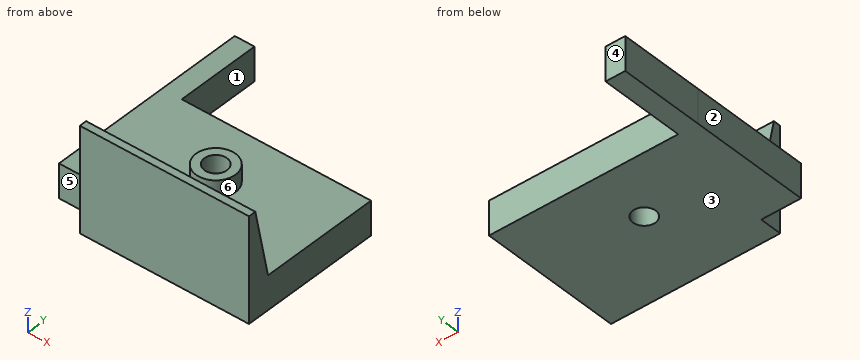
from build123d import *

# Parameters (mm, degrees)
F0_W      = 3.500263
F0_H      = 15
F1_DEPTH  = 6
F2_R      = 3.5
F2_R_2    = 2
F3_DEPTH  = 3
F3_FACE_R = 2
F4_DEPTH  = 25
F6_DEPTH  = 30


with BuildPart() as f1:
    # F0 (on Top) → F1 (new body)
    with BuildSketch(Plane.XY):
        with Locations((-35.299869, 28.75)):
            Rectangle(F0_W, F0_H)
        Polygon((-37.05, 0), (0, 0), (0, 21.25), (-33.549737, 21.25), (-37.05, 21.25), align=None)
    extrude(amount=F1_DEPTH)

    # F2 (on face) → F3 (join)
    with BuildSketch(Plane.XY.offset(6)):
        with Locations((-18.5, 10.75)):
            Circle(F2_R)
        with Locations((-18.5, 10.75)):
            Circle(F2_R_2, mode=Mode.SUBTRACT)
    extrude(amount=F3_DEPTH)

    # F3_face (on face) → F4 (cut)
    with BuildSketch(Plane(origin=(-18.5, 10.75, 6), x_dir=(1, 0, 0), z_dir=(0, 0, 1))):
        Circle(F3_FACE_R)
    extrude(amount=-F4_DEPTH, mode=Mode.SUBTRACT)

    # F5 (on face) → F6 (join)
    with BuildSketch(Plane.YZ):
        Polygon((-3.914129, 0), (0, 0), (0, 6), (-2.612495, 18.507209), (-3.914129, 18.507209), align=None)
    extrude(amount=-F6_DEPTH)


solid = f1.part
Check sheet for the modelled part. Datum: model origin and axes. Units: mm. Face numbers are marked on the shaded views. A direction names the side the tool comes from. Give positions to 0.01 mm unless a question says otherwise; leave off trailing zeros. Write each loop counter-clockwise with the first axis right and the second up, starting at its lowest first coordinate (ties: lowest second). Pieces come first, ordered by that corner, then holes. Notation, with made-up numbers: (38.5, 68.25) -> (70.5, 68.25) arc R15 ccw to (70.5, 95.25) -> close; hole circle Ø2 at (-31.5, -26). An arc over 180 degrees is marked (long way). Write item = value, one per line.
Item 1: Sectioned sample at B-B on y = 10.75. Record the boundary of the cut face in (x, z).
Output:
outline = (-37.05, 0) -> (-20.5, 0) -> (-20.5, 9) -> (-22, 9) -> (-22, 6) -> (-37.05, 6) -> close; (-16.5, 0) -> (0, 0) -> (0, 6) -> (-15, 6) -> (-15, 9) -> (-16.5, 9) -> close
Item 2: Release check for a two-part mould opening along Y. For the marked faces 3, 4, 5 and 6 record: +Y half, -Y half, draft (parallel to the pull), parting line (faces both ways), or undercut.
Output:
face_3 = draft
face_4 = +Y half
face_5 = -Y half
face_6 = undercut
Item 3: Scan lines: probe 1 along Y at (x, z) = (-18.5, 1.6); probe 2 along Z at (x, y) = (-32.5, 15.5); probe 3 along Y at (x, z) = (-21.5, 3.75). Record each from-to range of solid material in increasing order. Write a range as from..to.
Output:
probe_1 = -3.91..8.75, 12.75..21.25
probe_2 = 0..6
probe_3 = -3.91..21.25
Item 4: Gauge pin test, flat ends, axial feed: pin 1 (1 mm diameter, centred on x = -7.5, z = 9, fed in from +Y); pin 2 (5 mm diameter, centred on x = -10.5, z = 4.5, fed in from +Y); pin 3 (1.8 mm diameter, centred on x = -32.5, z = 3.5, fed in from -Y). Record the tip position at first contact, or that the pin passes through.
Output:
pin_1 = -0.52
pin_2 = 21.25
pin_3 = 0
Item 5: Sectioned sample at A-A on x = -18.5. Record the boundary of the cut face in (y, z), and give its area (3 significant figures).
Output:
outline = (-3.91, 0) -> (8.75, 0) -> (8.75, 9) -> (7.25, 9) -> (7.25, 6) -> (0, 6) -> (-2.61, 18.51) -> (-3.91, 18.51) -> close; (12.75, 0) -> (21.25, 0) -> (21.25, 6) -> (14.25, 6) -> (14.25, 9) -> (12.75, 9) -> close
area = 169 mm^2
Item 6: Tool access check on the marked faces 1 and 2. Record the directions out of +Z, -Z, +X, -X, +Y, -Y that give a thin tool (end or side, any length) a straight path to the whole face; none if there is none.
Output:
face_1 = +Z, -Z, +X, +Y
face_2 = +Z, -Z, -X, +Y, -Y
Item 7: Sectioned sample at C-C on z = 3.5. Record the boundary of the cut face in (x, y), and give its area (3 significant figures).
Output:
outline = (-37.05, 0) -> (-30, 0) -> (-30, -3.91) -> (0, -3.91) -> (0, 21.25) -> (-33.55, 21.25) -> (-33.55, 36.25) -> (-37.05, 36.25) -> close; hole circle Ø4 at (-18.5, 10.75)
area = 945 mm^2
Item 8: Sectioned sample at D-D on x = -10. Record the boundary of the cut face in (y, z), and give its area (3 significant figures).
Output:
outline = (-3.91, 0) -> (21.25, 0) -> (21.25, 6) -> (0, 6) -> (-2.61, 18.51) -> (-3.91, 18.51) -> close
area = 184 mm^2
